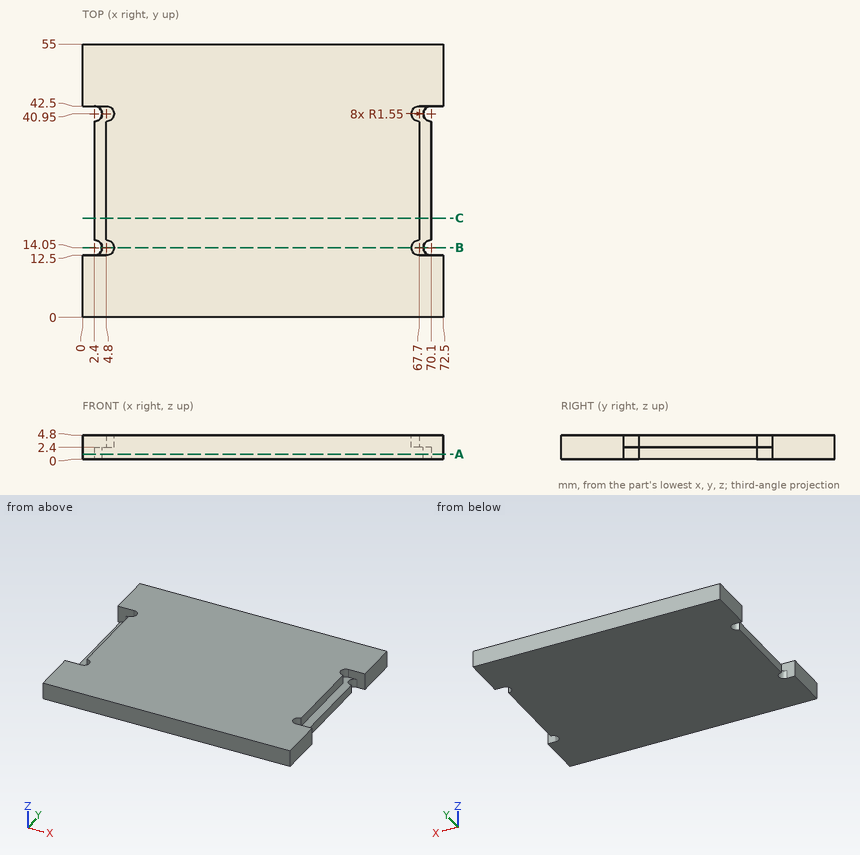
Design review of the part shown in the three views and the two pictorial views. Dimensions are in mm from the part's minimum x, y and z. Round coordinates to 2 decimals unless told otherwise and drop trailing zeros. Order: outer loops, then holes, each group sorted by start corner. A loop starts at its lowest first (then second) coordinate and runs counter-clockwise, first axis right, second up.
Item 1: For pin 1 (1.9 mm diameter, centred on y = 28, z = 0.5, fed in from -X); pin 2 (0.7 mm diameter, centred on y = 30.5, z = 3.5, fed in from -X); pin 3 (2 mm diameter, centred on x = 3.5, y = 35, fed in from +Z), all flat-tipped, find the tip position at first contact; note any pin that passes through.
Working result:
pin 1: stops at x = 2.4
pin 2: stops at x = 4.8
pin 3: stops at z = 2.4
Item 2: To check wall thickness, follow probe 1 along Y at (x, z) = (4.5, 4.3); probe 2 along X at (y, z) = (16, 1.75); probe 3 along X at (y, z) = (30.5, 4.3). State the ranges of each line that lie inside material, in increasing order.
Working result:
probe 1: y = 0 to 12.5, 42.5 to 55
probe 2: x = 2.4 to 70.1
probe 3: x = 4.8 to 67.7
Item 3: Add section C-C, the plane y = 20. State the section outline as (x, z) points.
Working result:
outline: (2.4, 0) - (70.1, 0) - (70.1, 2.4) - (67.7, 2.4) - (67.7, 4.8) - (4.8, 4.8) - (4.8, 2.4) - (2.4, 2.4) - close
Item 4: Add section A-A, the plane z = 1.05. State the section outline as (x, y) points.
Working result:
outline: (0, 0) - (72.5, 0) - (72.5, 12.5) - (70.1, 12.5) arc R1.55 cw to (70.1, 15.6) - (70.1, 39.4) arc R1.55 cw to (70.1, 42.5) - (72.5, 42.5) - (72.5, 55) - (0, 55) - (0, 42.5) - (2.4, 42.5) arc R1.55 cw to (2.4, 39.4) - (2.4, 15.6) arc R1.55 cw to (2.4, 12.5) - (0, 12.5) - close
Item 5: Add section B-B, the plane y = 14.05. State the section outline as (x, z) points, and give its area (3 significant figures).
Working result:
outline: (3.95, 0) - (68.55, 0) - (68.55, 2.4) - (66.15, 2.4) - (66.15, 4.8) - (6.35, 4.8) - (6.35, 2.4) - (3.95, 2.4) - close
area: 299 mm2
